Answer from the drawing. Dimensions are ordinates in mm from the lowest x, y and z of the part. A direction names the side the tool comes from. Coordinates: 2 decimals unless noted, no trailing zeros. Write each loop counter-clockwise with the first axis right and the second up, starting at its lowest first coordinate (ties: lowest second). Pieces come first, ordered by that corner, then holes.
(1) The part is cut by section B-B, the plane x = 10. Determine the outline of the cut face in (y, z) (1 decimal), and give its area (3 significant figures).
(2) Straight lines are drawn through the part: line 1 along Z through (x, y) = (13, 174); line 2 along Y through (x, z) = (30, 18) (1 decimal); line 3 along Y through (x, z) = (5, 21). For each, find the intervals that lie inside material, in ascending order.
(3) Determine the mould class of the marked faces 1, 2 and 3 for opening direction Y: pulls with the +Y half, pulls with the -Y half, needs draft (parallel to the pull), parting line crosses it, or undercut.
(4) The part is cut by section D-D, the plane x = 61. Determine the outline of the cut face in (y, z) (1 decimal), and give its area (3 significant figures).
(5) Which of the six approach directions +Z, -Z, +X, -X, +Y, -Y give full straight-line access (tool end or side, diameter ignored) to the marked faces 4, 5 and 6?
(6) The part is cut by section A-A, the plane z = 20. Determine the outline of the cut face in (x, y).
(7) The part is cut by section C-C, the plane y = 227.5. Determine the outline of the cut face in (x, z).
(8) Given pin 1 (12 mm diameter, centred on x = 60, y = 111, fed in from -Z); pin 2 (24.5 mm diameter, centred on x = 37, z = 14, fed in from +Y) (1 decimal); pin 3 (2 mm diameter, centred on x = 55.5, z = 69.5, fed in from +Y), each flat-ended and moving along its own axis, determine where each tip first touches the part or whether it passes through.
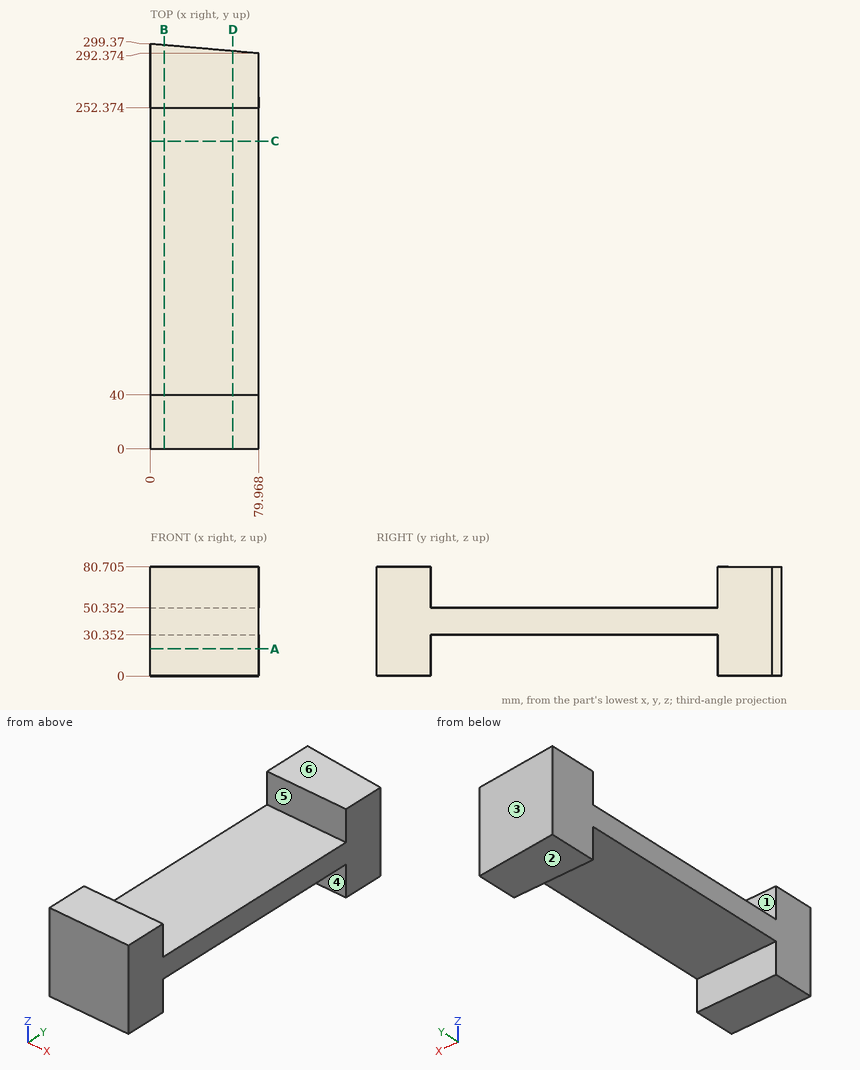
Computed:
1. outline: (0, 0) - (40, 0) - (40, 30.4) - (252.4, 30.4) - (252.4, 0) - (298.5, 0) - (298.5, 80.7) - (252.4, 80.7) - (252.4, 50.4) - (40, 50.4) - (40, 80.7) - (0, 80.7) - close
1. area: 11,200 mm2
2. line 1: z = 30.35 to 50.35
2. line 2: y = 0 to 40, 252.4 to 296.7
2. line 3: y = 0 to 40, 252.37 to 298.93
3. face 1: undercut
3. face 2: needs draft
3. face 3: pulls with the +Y half
4. outline: (0, 0) - (40, 0) - (40, 30.4) - (252.4, 30.4) - (252.4, 0) - (294, 0) - (294, 80.7) - (252.4, 80.7) - (252.4, 50.4) - (40, 50.4) - (40, 80.7) - (0, 80.7) - close
4. area: 10,800 mm2
5. face 4: -Z, +X, -X
5. face 5: +Z, +X, -X
5. face 6: +Z, +X, -X, +Y, -Y
6. outline: (0, 0) - (79.97, 0) - (79.97, 40) - (0, 40) - close; (0, 252.37) - (79.97, 252.37) - (79.97, 292.37) - (0, 299.37) - close
7. outline: (0, 30.35) - (79.97, 30.35) - (79.97, 50.35) - (0, 50.35) - close
8. pin 1: stops at z = 30.35
8. pin 2: stops at y = 297.2
8. pin 3: stops at y = 294.6
